from build123d import *

# Parameters (mm, degrees)
F0_W     = 76.2
F0_H     = 114.3
F1_DEPTH = 63.5
F2_W     = 69.85
F2_H     = 107.95
F3_DEPTH = 60.325
F4_R     = 2.54
F5_R     = 31.75
F6_DEPTH = 3.175
F7_R     = 3.175
F8_DEPTH = 3.175


with BuildPart() as f1:
    # F0 (on Top) → F1 (new body)
    with BuildSketch(Plane.XY):
        Rectangle(F0_W, F0_H)
    extrude(amount=F1_DEPTH)

    # F2 (on face) → F3 (cut)
    with BuildSketch(Plane.XY.offset(63.5)):
        Rectangle(F2_W, F2_H)
    extrude(amount=-F3_DEPTH, mode=Mode.SUBTRACT)

    # F4
    f4_edges = [f1.edges().sort_by_distance(p)[0] for p in [
        (34.925, 53.975, 33.3375),
        (34.925, -53.975, 33.3375),
        (-34.925, -53.975, 33.3375),
        (-34.925, 53.975, 33.3375),
        (38.1, -57.15, 31.75),
        (38.1, 57.15, 31.75),
        (-38.1, -57.15, 31.75),
        (-38.1, 57.15, 31.75),
        (-38.1, 0, 0),
        (0, 57.15, 0),
        (0, -57.15, 0),
        (38.1, 0, 0),
    ]]
    fillet(f4_edges, radius=F4_R)

    # F5 (on face) → F6 (cut, through all)
    with BuildSketch(Plane.XY.offset(3.175)):
        Circle(F5_R)
    extrude(amount=-F6_DEPTH, mode=Mode.SUBTRACT)

    # F7 (on face) → F8 (cut, through all)
    with BuildSketch(Plane.XY.offset(3.175)):
        with Locations((30.1625, 30.1625)):
            Circle(F7_R)
        with Locations((30.1625, -30.1625)):
            Circle(F7_R)
        with Locations((-30.1625, -30.1625)):
            Circle(F7_R)
        with Locations((-30.1625, 30.1625)):
            Circle(F7_R)
    extrude(amount=-F8_DEPTH, mode=Mode.SUBTRACT)


solid = f1.part
Design review of the part built by this model. Coordinates are the model's own, in mm. A direction names the side the tool comes from. Round coordinates to 2 decimals unless told otherwise and drop trailing zeros. Write each loop counter-clockwise with the first axis right and the second up, starting at its lowest first coordinate (ties: lowest second). Pieces come first, ordered by that corner, then holes.
Item 1: Wall thickness on L1, parallel to Y at x = 0, z = 34 (3 decimals); L2, parallel to X at y = -6, z = 21 (3 decimals); L3, parallel to Z at x = 26.5, y = 35 (3 decimals): over which ranges is each line inside the solid? List them lowest first.
Item 2: Consider section B-B on z = 26. Give the boundary of the cut face in (x, y) (3 decimals), and give its area (3 significant figures).
Item 3: For faces 5 (the cylindrical face through (-27.23, 28.95, 1.61)), 6 (the cylindrical face through (-34.16, 53.25, 32.92)), list the 3-axis set-ups (+Z, -Z, +X, -X, +Y, -Y) from which the entire face can be reached by the end or side of a thin tool; tool diameter is ignored.
Item 4: Draft analysis for pull direction X (two halves, no side actions). For faces 1 (the cylindrical face through (-37.376, 56.386, 33.447)), 2 (the flat face through (38.1, -1, 33)), 3 (the flat face through (0, 53.975, 34)), 4 (the flat face through (-32, -11, 3.175)), state which applies: released by +X, released by -X, zero draft, split by the parting line, or undercut.
Item 5: For pin 1 Ø10 at (x, y) = (-30.16, -30.16) entering from +Z; pin 2 Ø10 at (x, y) = (28, -18.5) entering from +Z (3 decimals), all flat-tipped, find the tip position at first contact; note any pin that passes through.
Item 6: Consider section A-A on x = 0. Give the boundary of the cut face in (y, z) (3 decimals).
Item 7: Consider section C-C on y = 0. Give the boundary of the cut face in (x, z) (3 decimals).
Check values:
1. L1: y = -57.15 to -53.975, 53.975 to 57.15
1. L2: x = -38.1 to -34.925, 34.925 to 38.1
1. L3: z = 0 to 3.175
2. outline: (-38.1, -54.61) arc R2.54 ccw to (-35.56, -57.15) - (35.56, -57.15) arc R2.54 ccw to (38.1, -54.61) - (38.1, 54.61) arc R2.54 ccw to (35.56, 57.15) - (-35.56, 57.15) arc R2.54 ccw to (-38.1, 54.61) - close; hole (-34.925, -51.435) arc R2.54 ccw to (-32.385, -53.975) - (32.385, -53.975) arc R2.54 ccw to (34.925, -51.435) - (34.925, 51.435) arc R2.54 ccw to (32.385, 53.975) - (-32.385, 53.975) arc R2.54 ccw to (-34.925, 51.435) - close
2. area: 1,170 mm2
3. face 5: +Z, -Z
3. face 6: +Z
4. face 1: released by -X
4. face 2: released by +X
4. face 3: undercut
4. face 4: undercut
5. pin 1: stops at z = 63.5
5. pin 2: stops at z = 3.175
6. outline: (-57.15, 2.54) arc R2.54 ccw to (-54.61, 0) - (-31.75, 0) - (-31.75, 3.175) - (-53.975, 3.175) - (-53.975, 63.5) - (-57.15, 63.5) - close; (31.75, 0) - (54.61, 0) arc R2.54 ccw to (57.15, 2.54) - (57.15, 63.5) - (53.975, 63.5) - (53.975, 3.175) - (31.75, 3.175) - close
7. outline: (-38.1, 2.54) arc R2.54 ccw to (-35.56, 0) - (-31.75, 0) - (-31.75, 3.175) - (-34.925, 3.175) - (-34.925, 63.5) - (-38.1, 63.5) - close; (31.75, 0) - (35.56, 0) arc R2.54 ccw to (38.1, 2.54) - (38.1, 63.5) - (34.925, 63.5) - (34.925, 3.175) - (31.75, 3.175) - close
